Source: CAD feature listing. Evaluate the final solid. Frame: model axes, mm. Give positions to 0.01 mm unless a question says otherwise; leave off trailing zeros. Loops run counter-clockwise (first coordinate to the right, second up) from the corner with the lowest first, then second, coordinate; pieces in that order, holes last. Notation, with made-up numbers: (23, -37) - (71, -37) arc R24 ccw to (71, 2) - close; hole circle Ø10 at (83, 52). An arc over 180 degrees is marked (long way). Write each question's results on one line, items separated by ' | '. Start each with the question number.
(1) Cut plane A-A on y = -1.75. Return the cut outline in (x, z).
(2) Contact query for flat-ended pins moving along their axis: pin 1 (5 mm diameter, centred on x = 8.5, y = -16, fed in from +Z); pin 2 (2 mm diameter, centred on x = 13, z = 14, fed in from -Y); pin 3 (2 mm diameter, centred on x = 3, y = -8.5, fed in from -Z). Output: stop coordinate, or through.
(3) Cut plane B-B on x = 6.25. Return the cut outline in (y, z).
(4) Material intervals for line 1 along Y through (x, z) = (7.75, 13.75); line 2 along Z through (x, y) = (7.75, -4.25); line 3 along Z through (x, y) = (13.75, -4.75), sorted ascending. Write a range as [from, to].
(5) Pull-direction query (Z, two-part tool) for faces 1 (the cylindrical face through (5.24, -1.18, 4.96)), 2 (the flat face through (14.5, -6, 19)), 3 (the cylindrical face through (7.4, -11.08, 19.56)); classes: pulls with the +Z half, pulls with the -Z half, needs draft (parallel to the pull), parting line crosses it, or undercut.
(6) Cut plane C-C on x = 8. Return the cut outline in (y, z).
(7) Cut plane D-D on z = 2.25. Return the cut outline in (x, y).
from build123d import *

# Parameters (mm, degrees)
BOSS_EXTRUDE1_DEPTH = 2.4
BOSS_EXTRUDE3_DEPTH = 20
FILLET2_R           = 2
SKETCH7_R           = 3.3
CUT_EXTRUDE1_DEPTH  = 34.346813941


with BuildPart() as part:
    # Sketch4 → Boss-Extrude1 (new body)
    with BuildSketch(Plane(origin=(0, 0, 0), x_dir=(1, 0, 0), z_dir=(0, 1, 0))):
        with BuildLine():
            Line((0, 0), (0, -20))
            ThreePointArc((0, -20), (7.299964439, -19.572220189), (14.5, -18.294736614))
            Line((14.5, -18.294736614), (14.5, 2.550031289))
            ThreePointArc((14.5, 2.550031289), (7.361261094, 0.642362285), (0, 0))
        make_face()
    extrude(amount=-BOSS_EXTRUDE1_DEPTH)

    # Sketch6 → Boss-Extrude3 (add)
    with BuildSketch(Plane(origin=(0, 0, 0), x_dir=(1, 0, 0), z_dir=(0, 1, 0))):
        with BuildLine():
            Line((0, -20), (0, -22.4))
            ThreePointArc((0, -22.4), (7.296255081, -21.988562256), (14.5, -20.759465695))
            Line((14.5, -20.759465695), (14.5, -18.294736614))
            ThreePointArc((14.5, -18.294736614), (7.299964439, -19.572220189), (0, -20))
        make_face()
    extrude(amount=-BOSS_EXTRUDE3_DEPTH)

    # Fillet2
    fillet2_edges = [part.edges().sort_by_distance(p)[0] for p in [
        (14.5, -1.2, -2.550031289),
        (0, -1.2, 0),
    ]]
    fillet(fillet2_edges, radius=FILLET2_R)

    # Sketch7 → Cut-Extrude1 (cut, through all)
    with BuildSketch(Plane(origin=(0, 0, 0), x_dir=(1, 0, 0), z_dir=(0, 1, 0))):
        with Locations(Location((7.25, -7.57807584, 0), (0, 0, 270))):
            Circle(SKETCH7_R)
    extrude(amount=-CUT_EXTRUDE1_DEPTH, mode=Mode.SUBTRACT)


solid = part.part
Ans:
1) outline: (0, 1.96) arc R2 ccw to (1.91, -0.04) arc R42.5 cw to (11.94, -1.71) arc R2 ccw to (14.5, 0.21) - (14.5, 20.76) arc R64.9 ccw to (0, 22.4) - close; hole circle Ø6.6 at (7.25, 7.58)
2) pin 1: z = 22.12 | pin 2: y = -2.4 | pin 3: z = 19.87
3) outline: (-20, 19.69) - (-2.4, 19.69) - (-2.4, 10.72) - (0, 10.72) - (0, 22.1) - (-20, 22.1) - close; (-2.4, -0.46) - (0, -0.46) - (0, 4.43) - (-2.4, 4.43) - close
4) line 1: [-2.4, 0] | line 2: [19.52, 21.94] | line 3: [18.47, 20.93]
5) face 1: undercut | face 2: needs draft | face 3: pulls with the -Z half
6) outline: (-20, 19.49) - (-2.4, 19.49) - (-2.4, 10.79) - (0, 10.79) - (0, 21.91) - (-20, 21.91) - close; (-2.4, -0.76) - (0, -0.76) - (0, 4.36) - (-2.4, 4.36) - close
7) outline: (0, -2.4) - (14.5, -2.4) - (14.5, 0) - (0, 0) - close
